Could you check a few things on this model? Use its own coordinates, in mm. Face numbers are marked on the shaded views. A direction names the side the tool comes from. Round coordinates to 2 decimals unless told otherwise and drop trailing zeros. Loops run counter-clockwise (first coordinate to the right, second up) from the corner with the lowest first, then second, coordinate; pieces in that order, holes last. Notation, with made-up numbers: (3.25, 35) -> (53.25, 35) arc R27 ccw to (53.25, 68) -> close; hole circle Ø1 at (34, 59.25). An arc over 180 degrees is marked (long way). Put each result on its own line as item: value. Start each with the question number.
1. Imagine slicing it at D-D, the plane z = -6. Please give me the cut outline in (x, y), and give its area (3 significant figures).
2. I need wall thicknesses on line 1 (Y direction, x = -7.5, z = 17); line 2 (Z direction, x = -22.5, y = 9); line 3 (X direction, y = 11.25, z = 2.5). Which ranges of each line are inside material? Lowest first, please. Write a range as [from, to].
3. I'm going to push flat-ended pins straight in: P1, Ø4, axis at y = 18, z = -1.5, coming from the +X side; P2, Ø4, axis at x = -8.5, y = 13.5, coming from the +Z side; P3, Ø12, axis at x = -9, y = 12, coming from the -Z side. Where does each tip first touch, or does it pass through?
4. Which directions (+Z, -Z, +X, -X, +Y, -Y) give clear straight access to the entire face, cutting with the end or side of a thin tool? Please do the marked faces 1 and 2.
5. Imagine slicing it at A-A, the plane y = 2.25. Please give me the cut outline in (x, z).
6. Imagine slicing it at B-B, the plane z = 6. Please give me the cut outline in (x, y).
7. Imagine slicing it at C-C, the plane x = -2.5. Please give me the cut outline in (y, z), and give its area (3 significant figures).
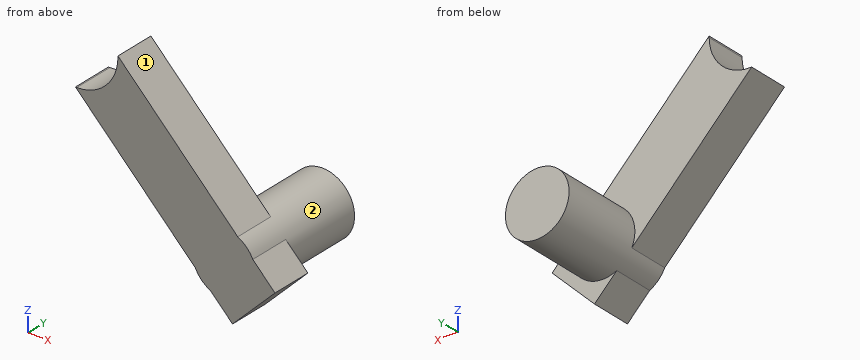
Autodesk Inventor part; units mm, degrees
ref_plane "YZ Plane" through (0, 0, 0) normal (1, 0, 0) x (0, 1, 0)
ref_plane "XZ Plane" through (0, 0, 0) normal (0, 1, 0) x (-1, 0, 0)
ref_plane "XY Plane" through (0, 0, 0) normal (0, 0, 1) x (1, 0, 0)
sketch "Sketch1" plane through (0, 0, 0) normal (0, 1, 0) x (-1, 0, 0)
  circle A0 centre (0.0391, 0.0653) radius 7.75
  line L0 (25.8724, 25.8987) -> (36.2057, 25.8987)
  line L1 (25.8724, 36.232) -> (25.8724, 25.8987)
  line L2 (36.2057, 25.8987) -> (-2.0324, -12.3395)
  line L3 (25.8724, 36.232) -> (-12.3657, -2.0061)
  line L4 (25.8724, 36.232) -> (79.9493, 36.232) construction
  line L5 (-12.3657, -2.0061) -> (-2.0324, -12.3395)
  point P0 (0, 0)
  point P1 (-53.1731, 12.2093)
  point P2 (3.379, -6.928)
  point P3 (-6.9543, 3.4053)
  point P4 (-3.3009, 7.0587)
  point P5 (7.0324, -3.2747)
  dimension "d0" = 15.5
  dimension "d1" = 135
extrude "Extrusion1" add sketch "Sketch1" along normal blind 10 contours A0 L3 L1 L0 L2 | A0 L2 L5 L3
extrude "Extrusion2" add sketch "Sketch1" along normal blind 30 contours A0 L2 L3 | L3 A0 | A0 L2
fillet "Fillet1" radius 10 1 edges at (-25.8724, 5, 25.8987)
properties part number "hjørner holder"
Entries:
1. outline: (-4.86, 0) -> (8.37, 0) -> (8.37, 10) -> (4.79, 10) -> (4.79, 30) -> (-4.86, 30) -> close
1. area: 325 mm^2
2. line 1: [0, 10]
2. line 2: [12.19, 32.86]
2. line 3: [-7.4, 7.32]
3. P1: x = 7.71
3. P2: z = 4.35
3. P3: z = -7.1
4. face 1: +Z, +X, +Y, -Y
4. face 2: +Y
5. outline: (-36.21, 25.9) -> (-7.03, -3.27) arc R7.75 ccw to (-3.38, -6.93) -> (2.03, -12.34) -> (12.37, -2.01) -> (6.95, 3.41) arc R7.75 ccw to (3.3, 7.06) -> (-25.87, 36.23) -> (-25.87, 35.9) arc R10 cw to (-35.87, 25.9) -> close
6. outline: (-16.31, 0) -> (4.95, 0) -> (4.95, 30) -> (-5.02, 30) -> (-5.02, 10) -> (-16.31, 10) -> close
7. outline: (0, -7.81) -> (10, -7.81) -> (10, -7.28) -> (30, -7.28) -> (30, 7.41) -> (10, 7.41) -> (10, 12.86) -> (0, 12.86) -> close
7. area: 501 mm^2
